Design review of the part built by this model. Coordinates are the model's own, in mm. Face numbers are marked on the shaded views. A direction names the side the tool comes from. Give positions to 0.01 mm unless a question says otherwise; leave off trailing zeros. Write each loop counter-clockwise with the first axis right and the second up, starting at its lowest first coordinate (ties: lowest second). Pieces come first, ordered by that corner, then holes. Notation, with made-up numbers: (24, 85.5) -> (28, 85.5) arc R17 cw to (28, 116.5) -> close; hole circle Ø3 at (6, 19). An arc over 180 degrees is marked (long way). Return JSON: item names as keys, results as strings. Group by question number.
from build123d import *

# Parameters (mm, degrees)
EXTRUDE_1_DEPTH = 10
FILLET_1_R      = 1
FILLET_2_R      = 2


with BuildPart() as part:
    # 草图1 → 凸台-拉伸1 (new body, symmetric)
    with BuildSketch(Plane.XY):
        Polygon((-15, 0), (0, 20), (15, 0), (25, 0), (25, 1), (15.5, 1), (0, 21.666666667), (-15.5, 1), (-25, 1), (-25, 0), align=None)
    extrude(amount=EXTRUDE_1_DEPTH, both=True)

    # 圆角1
    fillet_1_edges = [part.edges().sort_by_distance(p)[0] for p in [
        (0, 20, 0),
    ]]
    fillet(fillet_1_edges, radius=FILLET_1_R)

    # 圆角2
    fillet_2_edges = [part.edges().sort_by_distance(p)[0] for p in [
        (0, 21.666666667, 0),
    ]]
    fillet(fillet_2_edges, radius=FILLET_2_R)


solid = part.part
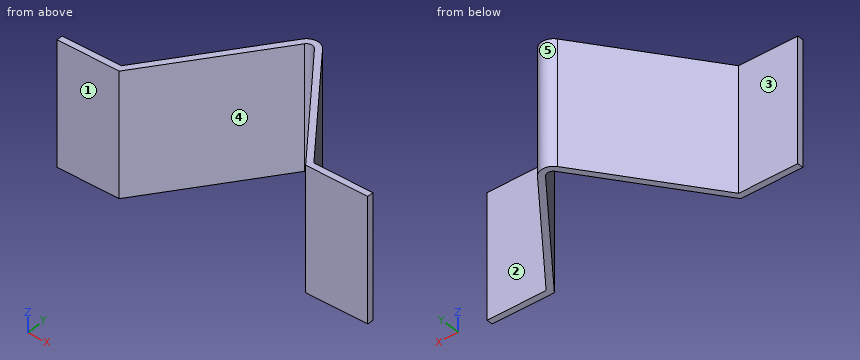
Q1. Insertion check: pin 1 (12 mm diameter, centred on x = 1.5, y = 12, fed in from +Z); pin 2 (4 mm diameter, centred on y = 9.5, z = 7, fed in from +X) (3 decimals); pin 3 (2 mm diameter, centred on x = -17, z = 0, fed in from +Y); pin 4 (1.5 mm diameter, centred on x = -13, z = -3, fed in from +Y). Each pin has a flat end and moves straight along its axis. Give the tip position at first contact, or say it passes through.
Q2. Take a section at C-C, the plane x = -16.5. Give the boundary of the cut face in (y, z).
Q3. Take a section at A-A, the plane y = 9. Give the boundary of the cut face in (x, z), plus the area to 3 significant figures.
Q4. Take a section at B-B, the plane z = 7.25. Give the boundary of the cut face in (x, y).
Q5. Tool access review of the marked faces 1 and 2: name each direction out of +Z, -Z, +X, -X, +Y, -Y from which nothing blocks a thin tool from reaching the whole face with its end or side.
Q6. Mouldability with a two-part tool opening along X and no side actions: class the marked faces 3, 4 and 5 as +X half, -X half, draft (parallel to the pull), parting line (faces both ways), or undercut.
Q7. For L1, parallel to Y at x = -20.5, z = -5.25; L2, parallel to X at y = 11.5, z = 2.5 (3 decimals); L3, parallel to X at y = 7.25, z = -4.25, list the stretches that pass through material, from the lowest coordinate up. Write a range as from..to.
Final values:
{
 "1": {"pin 1": "stops at z = 10", "pin 2": "stops at x = 10.625", "pin 3": "stops at y = 1", "pin 4": "stops at y = 5.33"},
 "2": {"outline": "(0, -10) -> (1, -10) -> (1, 10) -> (0, 10) -> close"},
 "3": {"outline": "(-9.5, -10) -> (-8.25, -10) -> (-8.25, 10) -> (-9.5, 10) -> close; (8.25, -10) -> (9.5, -10) -> (9.5, 10) -> (8.25, 10) -> close", "area": "50.0 mm²"},
 "4": {"outline": "(-25, 0) -> (-15, 0) -> (-0.8, 18.93) arc R1 cw to (0.8, 18.93) -> (15, 0) -> (25, 0) -> (25, 1) -> (15.5, 1) -> (1.6, 19.53) arc R2 ccw to (-1.6, 19.53) -> (-15.5, 1) -> (-25, 1) -> close"},
 "5": {"face 1": "+Z, -Z, +X, -X, -Y", "face 2": "+Z, -Z, +X, +Y"},
 "6": {"face 3": "draft", "face 4": "undercut", "face 5": "parting line"},
 "7": {"L1": "y = 0..1", "L2": "x = -7.625..-6.375, 6.375..7.625", "L3": "x = -10.81..-9.56, 9.56..10.81"}
}
